Source: CAD feature listing. Evaluate the final solid. Frame: model axes, mm. A direction names the side the tool comes from. Give positions to 0.01 mm unless a question says otherwise; leave off trailing zeros. One line per item, written item: value. Start each with the question number.
from build123d import *

# Parameters (mm, degrees)
F1_DEPTH     = 50.8
F2_R         = 1.5875
F3_T1_DEPTH  = 55.2235032041
F3_T3_DEPTH  = 55.9166206728
F4_T1_DEPTH  = 47.625
F4_T6_DEPTH  = 1.5875
F4_T12_DEPTH = 1.5875
F4_T18_DEPTH = 1.5875
F4_T24_DEPTH = 1.5875
F4_S29_W     = 1.5875
F4_S29_H     = 1.5875
F4_T30_DEPTH = 1.5875
F4_S35_W     = 1.5875
F4_S35_H     = 1.5875
F4_T36_DEPTH = 1.5875
F4_S41_W     = 1.5875
F4_S41_H     = 1.5875
F4_T42_DEPTH = 1.5875
F4_S47_W     = 1.5875
F4_S47_H     = 1.5875
F4_T48_DEPTH = 1.5875


# Not quite as in the source:
# - a fillet or chamfer that OpenCascade refuses, or shapes differently, is made with other operations: its cross-section is extruded or revolved along the edge and cut away or added


with BuildPart() as f1:
    # F0 (on Front) → F1 (new body)
    with BuildSketch(Plane.XZ):
        with BuildLine():
            Line((-18.2115888596, 55.5625), (-23.4099698747, -63.5))
            Line((-23.4099698747, -63.5), (-18.6474698747, -63.5))
            Line((-18.6474698747, -63.5), (-16.2727304656, -9.1095253353))
            ThreePointArc((-16.2727304656, -9.1095253353), (-13.3434580113, -2.6444832614), (-6.756796155, 0))
            Line((-6.756796155, 0), (0, 0))
            Line((0, 0), (0, 4.7625))
            ThreePointArc((0, 4.7625), (-8.9802561211, 8.4822438789), (-12.7, 17.4625))
            Line((-12.7, 17.4625), (-12.7, 55.5625))
            Line((-12.7, 55.5625), (-18.2115888596, 55.5625))
        make_face()
        with BuildLine():
            Line((0, 4.7625), (0, 0))
            Line((0, 0), (6.756796155, 0))
            ThreePointArc((6.756796155, 0), (13.3434580113, -2.6444832614), (16.2727304656, -9.1095253353))
            Line((16.2727304656, -9.1095253353), (18.6474698747, -63.5))
            Line((18.6474698747, -63.5), (23.4099698747, -63.5))
            Line((23.4099698747, -63.5), (18.2115888596, 55.5625))
            Line((18.2115888596, 55.5625), (12.7, 55.5625))
            Line((12.7, 55.5625), (12.7, 17.4625))
            ThreePointArc((12.7, 17.4625), (8.9802561211, 8.4822438789), (0, 4.7625))
        make_face()
    extrude(amount=F1_DEPTH)

    # F2
    f2_edges = [f1.edges().sort_by_distance(p)[0] for p in [
        (-20.810779, -50.8, -3.96875),
        (-21.02872, -50.8, -63.5),
        (-17.4601, -50.8, -36.304763),
        (-13.343458, -50.8, -2.644483),
        (0, -50.8, 0),
        (13.343458, -50.8, -2.644483),
        (17.4601, -50.8, -36.304763),
        (21.02872, -50.8, -63.5),
        (20.810779, -50.8, -3.96875),
        (15.455794, -50.8, 55.5625),
        (12.7, -50.8, 36.5125),
        (0, -50.8, 4.7625),
        (-12.7, -50.8, 36.5125),
        (-15.455794, -50.8, 55.5625),
        (-20.810779, 0, -3.96875),
        (-21.02872, 0, -63.5),
        (-17.4601, 0, -36.304763),
        (-13.343458, 0, -2.644483),
        (0, 0, 0),
        (13.343458, 0, -2.644483),
        (17.4601, 0, -36.304763),
        (21.02872, 0, -63.5),
        (20.810779, 0, -3.96875),
        (15.455794, 0, 55.5625),
        (12.7, 0, 36.5125),
        (0, 0, 4.7625),
        (-12.7, 0, 36.5125),
        (-15.455794, 0, 55.5625),
    ]]
    fillet(f2_edges, radius=F2_R)

    # F3: fillet of radius 1.5875 on 8 edges, made by hand

    # F3_s2 → F3_t1 (cut)
    with BuildSketch(Plane.XZ.offset(-2.2117516021)):
        with BuildLine():
            ThreePointArc((-18.2778772706, 54.0442457774), (-17.7896651949, 55.1217527898), (-16.6918882188, 55.5625))
            Line((-16.6918882188, 55.5625), (-18.2115888596, 55.5625))
            Line((-18.2115888596, 55.5625), (-18.2778772706, 54.0442457774))
        make_face()
        with BuildLine():
            ThreePointArc((16.6918882188, 55.5625), (17.7896651949, 55.1217527898), (18.2778772706, 54.0442457774))
            Line((18.2778772706, 54.0442457774), (18.2115888596, 55.5625))
            Line((18.2115888596, 55.5625), (16.6918882188, 55.5625))
        make_face()
    extrude(amount=F3_T1_DEPTH, mode=Mode.SUBTRACT)

    # F3_s4 → F3_t3 (cut)
    with BuildSketch(Plane.XZ.offset(-2.5583103364)):
        with BuildLine():
            ThreePointArc((-23.3376347919, -61.8432542226), (-22.8983985299, -63.0102769761), (-21.7516457401, -63.5))
            Line((-21.7516457401, -63.5), (-23.4099698747, -63.5))
            Line((-23.4099698747, -63.5), (-23.3376347919, -61.8432542226))
        make_face()
        with BuildLine():
            ThreePointArc((23.3376347919, -61.8432542226), (22.8983985299, -63.0102769761), (21.7516457401, -63.5))
            Line((21.7516457401, -63.5), (23.4099698747, -63.5))
            Line((23.4099698747, -63.5), (23.3376347919, -61.8432542226))
        make_face()
    extrude(amount=F3_T3_DEPTH, mode=Mode.SUBTRACT)

    # F4: fillet of radius 1.5875 on 4 edges, made by hand

    # F4_s2 → F4_t1 (cut)
    with BuildSketch(Plane.XZ.offset(1.5875)):
        with BuildLine():
            ThreePointArc((-14.2875, 55.5625), (-13.1649679849, 55.0975320151), (-12.7, 53.975))
            Line((-12.7, 53.975), (-12.7, 55.5625))
            Line((-12.7, 55.5625), (-14.2875, 55.5625))
        make_face()
        with BuildLine():
            ThreePointArc((12.7, 53.975), (13.1649679849, 55.0975320151), (14.2875, 55.5625))
            Line((14.2875, 55.5625), (12.7, 55.5625))
            Line((12.7, 55.5625), (12.7, 53.975))
        make_face()
        with BuildLine():
            ThreePointArc((-20.1671705155, -63.5), (-19.0693935395, -63.0592527898), (-18.5811814638, -61.9817457774))
            Line((-18.5811814638, -61.9817457774), (-18.6474698747, -63.5))
            Line((-18.6474698747, -63.5), (-20.1671705155, -63.5))
        make_face()
        with BuildLine():
            ThreePointArc((18.5811814638, -61.9817457774), (19.0693935395, -63.0592527898), (20.1671705155, -63.5))
            Line((20.1671705155, -63.5), (18.6474698747, -63.5))
            Line((18.6474698747, -63.5), (18.5811814638, -61.9817457774))
        make_face()
    extrude(amount=F4_T1_DEPTH, mode=Mode.SUBTRACT)


with BuildPart() as f4_tool4:
    # F4_s5 → F4_t6 (new body)
    with BuildSketch(Plane.XZ.offset(1.5875)):
        Polygon((20.1671705155, -61.9125), (18.5811814638, -61.9817457774), (18.6474698747, -63.5), (20.1671705155, -63.5), align=None)
    extrude(amount=-F4_T6_DEPTH)

    # F4_s7 → F4_t8 (revolve, cut)
    with BuildSketch(Plane(origin=(20.1671705155, -1.5875, -61.9125), x_dir=(0.6915130558, 0, 0.7223639621), z_dir=(-0.7223639621, 0, 0.6915130558))):
        with BuildLine():
            ThreePointArc((0, -1.5875), (1.5875, 0), (0, 1.5875))
            Line((0, 1.5875), (0, -1.5875))
        make_face()
    revolve(axis=Axis((20.1671705155, -1.5875, -61.9125), (0, 1, 0)), mode=Mode.SUBTRACT)


with BuildPart() as f1_1:
    add(f1.part)

    # F4_t3: cut F4_tool4
    add(f4_tool4.part, mode=Mode.SUBTRACT)


with BuildPart() as f4_tool10:
    # F4_s11 → F4_t12 (new body)
    with BuildSketch(Plane.XZ.offset(49.2125)):
        Polygon((20.1671705155, -61.9125), (18.5811814638, -61.9817457774), (18.6474698747, -63.5), (20.1671705155, -63.5), align=None)
    extrude(amount=F4_T12_DEPTH)

    # F4_s13 → F4_t14 (revolve, cut)
    with BuildSketch(Plane(origin=(20.1671705155, -49.2125, -61.9125), x_dir=(0.6915130558, 0, 0.7223639621), z_dir=(0.7223639621, 0, -0.6915130558))):
        with BuildLine():
            ThreePointArc((0, -1.5875), (1.5875, 0), (0, 1.5875))
            Line((0, 1.5875), (0, -1.5875))
        make_face()
    revolve(axis=Axis((20.1671705155, -49.2125, -61.9125), (0, -1, 0)), mode=Mode.SUBTRACT)


with BuildPart() as f1_2:
    add(f1_1.part)

    # F4_t9: cut F4_tool10
    add(f4_tool10.part, mode=Mode.SUBTRACT)


with BuildPart() as f4_tool16:
    # F4_s17 → F4_t18 (new body)
    with BuildSketch(Plane.XZ.offset(1.5875)):
        Polygon((-20.1671705155, -61.9125), (-20.1671705155, -63.5), (-18.6474698747, -63.5), (-18.5811814638, -61.9817457774), align=None)
    extrude(amount=-F4_T18_DEPTH)

    # F4_s19 → F4_t20 (revolve, cut)
    with BuildSketch(Plane(origin=(-20.1671705155, -1.5875, -61.9125), x_dir=(-0.6915130558, 0, 0.7223639621), z_dir=(-0.7223639621, 0, -0.6915130558))):
        with BuildLine():
            ThreePointArc((0, -1.5875), (1.5875, 0), (0, 1.5875))
            Line((0, 1.5875), (0, -1.5875))
        make_face()
    revolve(axis=Axis((-20.1671705155, -1.5875, -61.9125), (0, 1, 0)), mode=Mode.SUBTRACT)


with BuildPart() as f1_3:
    add(f1_2.part)

    # F4_t15: cut F4_tool16
    add(f4_tool16.part, mode=Mode.SUBTRACT)


with BuildPart() as f4_tool22:
    # F4_s23 → F4_t24 (new body)
    with BuildSketch(Plane.XZ.offset(49.2125)):
        Polygon((-20.1671705155, -61.9125), (-20.1671705155, -63.5), (-18.6474698747, -63.5), (-18.5811814638, -61.9817457774), align=None)
    extrude(amount=F4_T24_DEPTH)

    # F4_s25 → F4_t26 (revolve, cut)
    with BuildSketch(Plane(origin=(-20.1671705155, -49.2125, -61.9125), x_dir=(-0.6915130558, 0, 0.7223639621), z_dir=(0.7223639621, 0, 0.6915130558))):
        with BuildLine():
            ThreePointArc((0, -1.5875), (1.5875, 0), (0, 1.5875))
            Line((0, 1.5875), (0, -1.5875))
        make_face()
    revolve(axis=Axis((-20.1671705155, -49.2125, -61.9125), (0, -1, 0)), mode=Mode.SUBTRACT)


with BuildPart() as f1_4:
    add(f1_3.part)

    # F4_t21: cut F4_tool22
    add(f4_tool22.part, mode=Mode.SUBTRACT)


with BuildPart() as f4_tool28:
    # F4_s29 → F4_t30 (new body)
    with BuildSketch(Plane.YZ.offset(14.2875)):
        with Locations((-0.79375, 54.76875)):
            Rectangle(F4_S29_W, F4_S29_H)
    extrude(amount=-F4_T30_DEPTH)

    # F4_s31 → F4_t32 (revolve, cut)
    with BuildSketch(Plane(origin=(14.2875, -1.5875, 53.975), x_dir=(0, -0.7071067812, -0.7071067812), z_dir=(0, 0.7071067812, -0.7071067812))):
        with BuildLine():
            ThreePointArc((0, -1.5875), (1.5875, 0), (0, 1.5875))
            Line((0, 1.5875), (0, -1.5875))
        make_face()
    revolve(axis=Axis((14.2875, -1.5875, 53.975), (-1, 0, 0)), mode=Mode.SUBTRACT)


with BuildPart() as f1_5:
    add(f1_4.part)

    # F4_t27: cut F4_tool28
    add(f4_tool28.part, mode=Mode.SUBTRACT)


with BuildPart() as f4_tool34:
    # F4_s35 → F4_t36 (new body)
    with BuildSketch(Plane.YZ.offset(14.2875)):
        with Locations((-50.00625, 54.76875)):
            Rectangle(F4_S35_W, F4_S35_H)
    extrude(amount=-F4_T36_DEPTH)

    # F4_s37 → F4_t38 (revolve, cut)
    with BuildSketch(Plane(origin=(14.2875, -49.2125, 53.975), x_dir=(0, 0.7071067812, -0.7071067812), z_dir=(0, 0.7071067812, 0.7071067812))):
        with BuildLine():
            ThreePointArc((0, -1.5875), (1.5875, 0), (0, 1.5875))
            Line((0, 1.5875), (0, -1.5875))
        make_face()
    revolve(axis=Axis((14.2875, -49.2125, 53.975), (-1, 0, 0)), mode=Mode.SUBTRACT)


with BuildPart() as f1_6:
    add(f1_5.part)

    # F4_t33: cut F4_tool34
    add(f4_tool34.part, mode=Mode.SUBTRACT)


with BuildPart() as f4_tool40:
    # F4_s41 → F4_t42 (new body)
    with BuildSketch(Plane.XY.offset(53.975)):
        with Locations((-13.49375, -0.79375)):
            Rectangle(F4_S41_W, F4_S41_H)
    extrude(amount=F4_T42_DEPTH)

    # F4_s43 → F4_t44 (revolve, cut)
    with BuildSketch(Plane(origin=(-14.2875, -1.5875, 53.975), x_dir=(-0.7071067812, -0.7071067812, 0), z_dir=(-0.7071067812, 0.7071067812, 0))):
        with BuildLine():
            ThreePointArc((0, -1.5875), (1.5875, 0), (0, 1.5875))
            Line((0, 1.5875), (0, -1.5875))
        make_face()
    revolve(axis=Axis((-14.2875, -1.5875, 53.975), (0, 0, 1)), mode=Mode.SUBTRACT)


with BuildPart() as f1_7:
    add(f1_6.part)

    # F4_t39: cut F4_tool40
    add(f4_tool40.part, mode=Mode.SUBTRACT)


with BuildPart() as f4_tool46:
    # F4_s47 → F4_t48 (new body)
    with BuildSketch(Plane.XY.offset(53.975)):
        with Locations((-13.49375, -50.00625)):
            Rectangle(F4_S47_W, F4_S47_H)
    extrude(amount=F4_T48_DEPTH)

    # F4_s49 → F4_t50 (revolve, cut)
    with BuildSketch(Plane(origin=(-14.2875, -49.2125, 53.975), x_dir=(-0.7071067812, 0.7071067812, 0), z_dir=(0.7071067812, 0.7071067812, 0))):
        with BuildLine():
            ThreePointArc((0, -1.5875), (1.5875, 0), (0, 1.5875))
            Line((0, 1.5875), (0, -1.5875))
        make_face()
    revolve(axis=Axis((-14.2875, -49.2125, 53.975), (0, 0, 1)), mode=Mode.SUBTRACT)


with BuildPart() as f1_8:
    add(f1_7.part)

    # F4_t45: cut F4_tool46
    add(f4_tool46.part, mode=Mode.SUBTRACT)


solid = f1_8.part
1. Draft query along X for faces 1 (the cylindrical face through (-20.393, -0.477, -4.771)), 2 (the cylindrical face through (17.895, -50.323, -35.896)), 3 (the flat face through (16, -25, 55.562)). Return one class per face: pulls with the +X half, pulls with the -X half, needs draft (parallel to the pull), parting line crosses it, or undercut.
2. Set-up query: faces 4 (the flat face through (12.7, -25, 36)), 5 (the cylindrical face through (-17.86, -50.32, -35.16)), 6 (the cylindrical face through (17.895, -0.477, -35.896)), 7 (the flat face through (-17.443, -25.067, -35.916)). Return all of +Z, -Z, +X, -X, +Y, -Y with unobstructed straight access to the full face (end or side cutting, diameter ignored); none if empty.
3. Contact query for flat-ended pins moving along their axis: pin 1 Ø18.5 at (y, z) = (-17.5, 33.5) entering from +X; pin 2 Ø4 at (y, z) = (-24.5, -31) entering from -X; pin 3 Ø3 at (y, z) = (-13.5, -48) entering from +X. Output: stop coordinate, or through.
4. Ray query, L1, parallel to X at y = -16.5, z = 21; L2, parallel to X at y = -22, z = -24; L3, parallel to Z at x = -3, y = -27.5. Return the intervals inside material, ascending.
Data:
1. face 1: pulls with the -X half
1. face 2: undercut
1. face 3: needs draft
2. face 4: +Z, +Y, -Y
2. face 5: -Z, -Y
2. face 6: -Z, +Y
2. face 7: -Z, +Y, -Y
3. pin 1: stops at x = 19.58
3. pin 2: stops at x = -22.08
3. pin 3: stops at x = 22.8
4. L1: x = -19.72 to -12.7, 12.7 to 19.72
4. L2: x = -21.69 to -16.92, 16.92 to 21.69
4. L3: z = 0 to 5.12
